```python
from build123d import *

# Parameters (mm, degrees)
SKETCH1_R               = 2.667
BOSS_EXTRUDE1_DEPTH     = 6.35
SKETCH3_R               = 6.35
BOSS_EXTRUDE2_DEPTH     = 3.81
SKETCH4_R               = 4.7625
BOSS_EXTRUDE3_DEPTH     = 3.81
SKETCH5_R               = 6.35
SKETCH5_R_2             = 2.667
SKETCH5_R_3             = 5.08
SKETCH5_R_4             = 2.723974981
BOSS_EXTRUDE4_DEPTH     = 7.62
SKETCH6_W               = 54.822055163
SKETCH6_H               = 25.4
CUT_EXTRUDE2_DEPTH      = 10.414
CUT_EXTRUDE2_DEPTH_BACK = 156.972


with BuildPart() as part:
    # Sketch1 → Boss-Extrude1 (new body)
    with BuildSketch(Plane(origin=(0, 0, 0), x_dir=(-1, 0, 0), z_dir=(0, 1, 0))):
        with BuildLine():
            Line((132.859114436, 54.06756661), (1.925518385, 21.422154602))
            ThreePointArc((1.925518385, 21.422154602), (0.538452686, 20.521383604), (0, 18.957603457))
            Line((0, 18.957603457), (0, 3.251051746))
            ThreePointArc((0, 3.251051746), (0.976219853, 1.249504432), (3.154481615, 0.786500601))
            Line((3.154481615, 0.786500601), (135.868185597, 33.875743365))
            ThreePointArc((135.868185597, 33.875743365), (137.061865325, 33.884273203), (138.127619437, 33.346581632))
            ThreePointArc((138.127619437, 33.346581632), (145.587943549, 32.789337046), (148.401377862, 39.7212592))
            Line((148.401377862, 39.7212592), (145.116412217, 52.896536778))
            ThreePointArc((145.116412217, 52.896536778), (144.215641219, 54.283602477), (142.651861072, 54.822055163))
            Line((142.651861072, 54.822055163), (139.003930584, 54.822055163))
            ThreePointArc((139.003930584, 54.822055163), (135.908449262, 54.632727415), (132.859114436, 54.06756661))
        make_face()
        with Locations((142.24, 38.185055163)):
            Circle(SKETCH1_R, mode=Mode.SUBTRACT)
        with Locations((27.94, 12.785055202)):
            Circle(SKETCH1_R, mode=Mode.SUBTRACT)
        with Locations((104.14, 38.185055202)):
            Circle(SKETCH1_R, mode=Mode.SUBTRACT)
    boss_extrude1 = extrude(amount=-BOSS_EXTRUDE1_DEPTH)

    # Sketch3 → Boss-Extrude2 (add)
    with BuildSketch(Plane(origin=(0, -6.35, 0), x_dir=(-1, 0, 0), z_dir=(0, -1, 0))):
        with Locations((42.976982051, -23.804158196)):
            Circle(SKETCH3_R)
        with Locations((79.945249222, -33.021382418)):
            Circle(SKETCH3_R)
        with Locations((119.378067538, -42.853088255)):
            Circle(SKETCH3_R)
        with Locations((62.693391209, -28.720011114)):
            Circle(SKETCH3_R)
        with BuildLine():
            Line((0, -13.010825767), (0, -16.16304218))
            ThreePointArc((0, -16.16304218), (0.057532424, -16.700587281), (0.227523413, -17.213780985))
            ThreePointArc((0.227523413, -17.213780985), (12.35871488, -14.586933973), (0.227523413, -11.960086962))
            ThreePointArc((0.227523413, -11.960086962), (0.057532424, -12.473280666), (0, -13.010825767))
        make_face()
    boss_extrude2 = extrude(amount=BOSS_EXTRUDE2_DEPTH)

    # Sketch4 → Boss-Extrude3 (add)
    with BuildSketch(Plane.XZ.offset(10.16)):
        with Locations((-6.00871488, 14.586933973)):
            Circle(SKETCH4_R)
        with Locations((-42.976982051, 23.804158196)):
            Circle(SKETCH4_R)
        with Locations((-62.693391209, 28.720011114)):
            Circle(SKETCH4_R)
        with Locations((-79.945249222, 33.021382418)):
            Circle(SKETCH4_R)
        with Locations((-119.378067538, 42.853088255)):
            Circle(SKETCH4_R)
    boss_extrude3 = extrude(amount=BOSS_EXTRUDE3_DEPTH)

    # Sketch5 → Boss-Extrude4 (add)
    with BuildSketch(Plane.XZ.offset(6.35)):
        with Locations((-142.24, 38.185055163)):
            Circle(SKETCH5_R)
        with Locations((-142.24, 38.185055163)):
            Circle(SKETCH5_R_2, mode=Mode.SUBTRACT)
        with Locations((-27.94, 12.785055202)):
            Circle(SKETCH5_R_3)
        with Locations((-27.94, 12.785055202)):
            Circle(SKETCH5_R_4, mode=Mode.SUBTRACT)
        with BuildLine():
            Line((-105.580163175, 43.777970545), (-105.715311414, 41.562252701))
            ThreePointArc((-105.715311414, 41.562252701), (-105.443232026, 40.931048752), (-104.773674962, 40.775681582))
            ThreePointArc((-104.773674962, 40.775681582), (-101.589970205, 37.403878498), (-106.115998075, 36.393876649))
            ThreePointArc((-106.115998075, 36.393876649), (-106.757692083, 36.64019843), (-107.336634242, 36.269696613))
            Line((-107.336634242, 36.269696613), (-108.465736097, 34.358466745))
            ThreePointArc((-108.465736097, 34.358466745), (-108.561892576, 33.849199875), (-108.310080465, 33.396221428))
            ThreePointArc((-108.310080465, 33.396221428), (-98.068500487, 36.325110669), (-104.912246263, 44.487922463))
            ThreePointArc((-104.912246263, 44.487922463), (-105.374571656, 44.25371306), (-105.580163175, 43.777970545))
        make_face()
    boss_extrude4 = extrude(amount=BOSS_EXTRUDE4_DEPTH)

    # Mirror6: Boss-Extrude1, Boss-Extrude2, Boss-Extrude3, Boss-Extrude4 across plane
    add(boss_extrude1.mirror(Plane(origin=(-139.003930584, 0, 29.422055163), x_dir=(0, 0, 1), z_dir=(0, -1, 0))))
    add(boss_extrude2.mirror(Plane(origin=(-139.003930584, 0, 29.422055163), x_dir=(0, 0, 1), z_dir=(0, -1, 0))))
    add(boss_extrude3.mirror(Plane(origin=(-139.003930584, 0, 29.422055163), x_dir=(0, 0, 1), z_dir=(0, -1, 0))))
    add(boss_extrude4.mirror(Plane(origin=(-139.003930584, 0, 29.422055163), x_dir=(0, 0, 1), z_dir=(0, -1, 0))))

    # Sketch6 → Cut-Extrude2 (cut, two sides)
    with BuildSketch(Plane(origin=(0, 0, 0), x_dir=(0, 0, -1), z_dir=(1, 0, 0))) as cut_extrude2_sk:
        with Locations((-27.411027582, -12.7)):
            Rectangle(SKETCH6_W, SKETCH6_H)
    extrude(amount=CUT_EXTRUDE2_DEPTH, mode=Mode.SUBTRACT)
    extrude(cut_extrude2_sk.sketch, amount=-CUT_EXTRUDE2_DEPTH_BACK, mode=Mode.SUBTRACT)


solid = part.part
```
Read the model definition and answer for the solid it produces. Units are mm, in the model's axes. A direction names the side the tool comes from. Round coordinates to 2 decimals unless told otherwise and drop trailing zeros. Loops run counter-clockwise (first coordinate to the right, second up) from the corner with the lowest first, then second, coordinate; pieces in that order, holes last. Notation, with made-up numbers: (-2.5, 78) -> (14.5, 78) arc R14 cw to (14.5, 97) -> close; hole circle Ø6 at (79.5, -33). An arc over 180 degrees is marked (long way). One line per item, written item: value.
1) Flat-ended cylindrical pins translate along their axes: P1, Ø5, axis at x = -30, z = 25.5, coming from the +Y side; P2, Ø2, axis at x = -107, y = 3, coming from the +Z side; P3, Ø6, axis at x = -72, y = 11.5, coming from the +Z side. Find the tip coordinate at first contact, or state that the pin passes through.
Answer list:
P1: stops at y = 6.35
P2: stops at z = 47.87
P3: stops at z = 36.58
2) For faces 5 (the face through (-141, 3, 54.822)), 6 (the face through (-7.041, 12.038, 9.938)), determine the directions among +Z, -Z, +X, -X, +Y, -Y from which every point of the face is accessible in a straight line to the end or side of a thin tool.
Answer list:
face 5: +Z, +X, -X, +Y, -Y
face 6: +Y
3) The mould has two halves that part along X. Classify faces 1 (the face through (-42.2, 8.2, 17.5)), 2 (the face through (-146.78, 3.13, 46.22)), 3 (the face through (-98.12, 10.11, 36.16)), 4 (the face through (-68.309, 3.131, 37.973)): pulls with the +X half, pulls with the -X half, needs draft (parallel to the pull), parting line crosses it, or undercut.
Answer list:
face 1: undercut
face 2: pulls with the -X half
face 3: undercut
face 4: pulls with the +X half
4) A cutting plane is placed at B-B (x = -91.5). Determine the outline of the cut face in (y, z).
Answer list:
outline: (0, 22.81) -> (6.35, 22.81) -> (6.35, 43.76) -> (0, 43.76) -> close
5) A cutting plane is placed at A-A (x = -27.94). Determine the outline of the cut face in (y, z), and give its area (3 significant figures).
Answer list:
outline: (0, 6.97) -> (6.35, 6.97) -> (6.35, 7.71) -> (13.97, 7.71) -> (13.97, 10.06) -> (6.35, 10.06) -> (6.35, 10.12) -> (0, 10.12) -> close; (0, 15.45) -> (6.35, 15.45) -> (6.35, 15.51) -> (13.97, 15.51) -> (13.97, 17.87) -> (6.35, 17.87) -> (6.35, 27.91) -> (0, 27.91) -> close
area: 135 mm²
6) Consider L1, parallel to Z at x = -142.24, y = 3.25; L2, parallel to Y at x = -29, z = 26; L3, parallel to Z at x = -104.14, y = 4.75. Determine where each line is inside the solid, lowest interval first. Write a range as [from, to].
Answer list:
L1: z = [31.84, 35.52], [40.85, 54.82]
L2: y = [0, 6.35]
L3: z = [25.97, 35.52], [40.85, 46.91]
